```python
from build123d import *

# Parameters (mm, degrees)
F0_R     = 49.4170811362
F1_DEPTH = 7


with BuildPart() as f1:
    # F0 (on Top) → F1 (new body)
    with BuildSketch(Plane.XY):
        with BuildLine():
            add(Edge.make_bspline(
                [(0, 94.3807365658), (-0.0119379338, 95.2269886433), (-0.0118946907, 96.0715546279), (0, 96.9142982709)],
                knots=[0.5, 0.5, 0.5, 0.5, 0.5105644323, 0.5105644323, 0.5105644323, 0.5105644323], degree=3))
            Line((0, 94.3807365658), (0, 96.9142982709))
        make_face()
        with BuildLine():
            Line((0, 96.9142982709), (0, 94.3807365658))
            add(Edge.make_bspline(
                [(65.0650430471, 0), (27.9678273946, 10.5000054464), (0.565005932, 54.3287935629), (0, 94.3807365658)],
                knots=[0, 0, 0, 0, 0.5, 0.5, 0.5, 0.5], degree=3))
            add(Edge.make_bspline(
                [(65.0650430471, 0), (81.994375859, 14.4372666979), (122.6522566992, 31.9710162807), (165.9505028095, 15.6042415748), (181.7901432514, 0)],
                knots=[0, 0, 0, 0, 0.4993848001, 1, 1, 1, 1], degree=3))
            add(Edge.make_bspline(
                [(298.5152434558, 0), (281.5859106439, 14.4372666979), (240.9280298036, 31.9710162807), (197.6297836934, 15.6042415748), (181.7901432514, 0)],
                knots=[0, 0, 0, 0, 0.4993848001, 1, 1, 1, 1], degree=3))
            add(Edge.make_bspline(
                [(298.5152434558, 0), (335.6124591082, 10.5000054464), (390.4181020334, 98.1575816793), (337.8724828362, 170.7077774581), (298.5152434558, 188.7614731316)],
                knots=[0, 0, 0, 0, 0.5, 1, 1, 1, 1], degree=3))
            add(Edge.make_bspline(
                [(298.5152434558, 188.7614731316), (304.9228074129, 179.3974646966), (323.9386038821, 151.6077961536), (253.2731908086, 154.7519554988), (206.4191997051, 156.8366587162)],
                knots=[0, 0, 0, 0, 0.336960062, 1, 1, 1, 1], degree=3))
            Line((206.4191997051, 156.8366587162), (206.4191997051, 188.7614731316))
            Line((206.4191997051, 188.7614731316), (199.0741193295, 174.9168634415))
            Line((199.0741193295, 174.9168634415), (181.7901432514, 174.9168634415))
            Line((181.7901432514, 174.9168634415), (164.5061671734, 174.9168634415))
            Line((164.5061671734, 174.9168634415), (157.1610867977, 188.7614731316))
            Line((157.1610867977, 188.7614731316), (157.1610867977, 156.8366587162))
            add(Edge.make_bspline(
                [(65.0650430471, 188.7614731316), (58.65747909, 179.3974646966), (39.6416826207, 151.6077961536), (110.3070956942, 154.7519554988), (157.1610867977, 156.8366587162)],
                knots=[0, 0, 0, 0, 0.336960062, 1, 1, 1, 1], degree=3))
            add(Edge.make_bspline(
                [(0, 96.9142982709), (0.551064605, 135.9574482655), (26.5393774454, 171.0892315481), (65.0650430471, 188.7614731316)],
                knots=[0.5105644323, 0.5105644323, 0.5105644323, 0.5105644323, 1, 1, 1, 1], degree=3))
        make_face()
        with Locations((181.7901432514, 87.6324102283)):
            Circle(F0_R, mode=Mode.SUBTRACT)
    extrude(amount=F1_DEPTH)


solid = f1.part
```
Can you work these out from the model? Positions are in its coordinate system, mm. A direction names the side the tool comes from. Round coordinates to 2 decimals unless told otherwise and drop trailing zeros. Return JSON: item names as keys, results as strings. Group by question number.
1. Will these pins go through, and if not, where does the flat tip stop? pin 1 (4 mm diameter, centred on y = 35, z = 4.5, fed in from -X); pin 2 (4 mm diameter, centred on y = 85, z = 1.5, fed in from -X); pin 3 (4 mm diameter, centred on x = 71.5, z = 5, fed in from -Y); pin 4 (3 mm diameter, centred on x = 212, y = 154, fed in from -Z).
2. I need wall thicknesses on line 1 (X direction, y = 11.5, z = 2); line 2 (Y direction, x = 208, z = 1.5); line 3 (Y direction, x = 304, z = 2.75). Which ranges of each line are inside material? Lowest first, please. Write a range as [from, to].
3. Which directions (+Z, -Z, +X, -X, +Y, -Y) give clear straight access to the entire face, cutting with the end or side of a thin tool? Please do faces 3 (the face through (160.885, 181.742, 3.451)), 4 (the face through (198, 33, 0)).
4. We'd pull the mould along X, two halves only. Please class faces 1 (the face through (157.161, 173, 3)), 2 (the face through (198, 33, 7)): released by +X, released by -X, zero draft, split by the parting line, or undercut.
Output values:
{
 "1": {"pin 1": "x = 18.24", "pin 2": "x = 0.4", "pin 3": "y = 3.59", "pin 4": "z = 0"},
 "2": {"line 1": "[42, 81.34], [166.99, 196.59], [282.24, 321.58]", "line 2": "[17.26, 45.74], [129.53, 156.77]", "line 3": "[1.82, 161.01], [180.44, 186.08]"},
 "3": {"face 3": "+Z, -Z, +Y", "face 4": "-Z, +X, -X, +Y, -Y"},
 "4": {"face 1": "undercut", "face 2": "zero draft"}
}
